```python
from build123d import *

# Parameters (mm, degrees)
F0_W      = 129.2205303907
F0_H      = 41.7168587446
F1_DEPTH  = 152.4
F2_W      = 73.6317485571
F2_H      = 16.954690218
F2_W_2    = 73.8739818335
F2_H_2    = 16.7124718428
F3_DEPTH  = 25.4
F5_DEPTH  = 41.7178587446
F6_W      = 73.389545083
F6_H      = 15.5014246702
F7_DEPTH  = 25.4
F8_W      = 72.4207013845
F8_H      = 15.017002821
F9_DEPTH  = 25.4
F11_DEPTH = 75.7919326425
F13_DEPTH = 105.4396703839
F15_DEPTH = 137.5292986631


with BuildPart() as f1:
    # F0 (on Front) → F1 (new body)
    with BuildSketch(Plane.XZ):
        with Locations((-0.3052428365, -6.4101442695)):
            Rectangle(F0_W, F0_H)
    extrude(amount=F1_DEPTH)

    # F2 (on face) → F3 (cut)
    with BuildSketch(Plane.XY.offset(14.4482851028)):
        with Locations((1.6954615712, -25.9895175695)):
            Rectangle(F2_W, F2_H)
        with Locations((1.8165782094, -58.0823048949)):
            Rectangle(F2_W_2, F2_H_2)
    extrude(amount=-F3_DEPTH, mode=Mode.SUBTRACT)

    # F4 (on face) → F5 (cut, through all)
    with BuildSketch(Plane.XY.offset(14.4482851028)):
        Polygon((64.3050223589, 0), (0, 0), (64.3050223589, -25.4777166992), align=None)
        Polygon((-64.9155080318, 0), (-64.9155080318, -29.2058624327), (0, 0), align=None)
    extrude(amount=-F5_DEPTH, mode=Mode.SUBTRACT)

    # F6 (on face) → F7 (cut)
    with BuildSketch(Plane.XY.offset(14.4482851028)):
        with Locations((1.5743598342, -95.0192883611)):
            Rectangle(F6_W, F6_H)
    extrude(amount=-F7_DEPTH, mode=Mode.SUBTRACT)

    # F8 (on face) → F9 (cut)
    with BuildSketch(Plane.XY.offset(14.4482851028)):
        with Locations((1.0899379849, -126.5065521002)):
            Rectangle(F8_W, F8_H)
    extrude(amount=-F9_DEPTH, mode=Mode.SUBTRACT)

    # F10 (on face) → F11 (cut)
    with BuildSketch(Plane.XY.offset(14.4482851028)):
        Polygon((64.3050223589, -25.4777166992), (50.9865237329, -20.2009137), (50.9865237329, -152.4), align=None)
        Polygon((64.3050223589, -25.4777166992), (50.9865237329, -152.4), (64.3050223589, -152.4), align=None)
    extrude(amount=-F11_DEPTH, mode=Mode.SUBTRACT)

    # F12 (on face) → F13 (cut)
    with BuildSketch(Plane.XY.offset(14.4482851028)):
        Polygon((-45.9601895189, -152.4), (-45.9601895189, -20.677755026), (-64.9155080318, -29.2058624327), (-64.9155080318, -152.4), align=None)
    extrude(amount=-F13_DEPTH, mode=Mode.SUBTRACT)

    # F14 (on face) → F15 (cut)
    with BuildSketch(Plane.XY.offset(14.4482851028)):
        Polygon((0, 0), (-22.9800947595, -10.338877513), (25.4932618665, -10.338877513), align=None)
    extrude(amount=-F15_DEPTH, mode=Mode.SUBTRACT)


solid = f1.part
```
Model file for the job. Use its own axes, mm. A direction names the side the tool comes from. Round coordinates to 2 decimals unless told otherwise and drop trailing zeros. Write each loop counter-clockwise with the first axis right and the second up, starting at its lowest first coordinate (ties: lowest second). Pieces come first, ordered by that corner, then holes. Notation, with made-up numbers: (73.25, 28) - (111.25, 28) arc R14 ccw to (111.25, 39) - close; hole circle Ø3 at (-18.5, 49.25). An arc over 180 degrees is marked (long way). Use CSV: the item, a comma, the result in double quotes. Start each with the question number.
Item 1: Band-saw the part on A-A (z = -3). Write the cut outline in (x, y), and give its area (3 significant figures).
Item 2: Drill centre lines: L1, parallel to Y at x = -7.5, z = -1; L2, parallel to Y at x = -27, z = -6; L3, parallel to X at y = -24, z = 11.5. Where is each one in solid material? Low to high. Write a range as [from, to].
Item 3: Pin check, flat tips, straight feed: P1, Ø12, axis at x = -8, y = -126, coming from the +Z side; P2, Ø12.5, axis at x = 2.5, z = 4, coming from the +Y side; P3, Ø10, axis at x = 10, z = -6.5, coming from the +Y side. Stop position of each tip, or through.
Item 4: Band-saw the part on B-B (x = 20). Write the cut outline in (y, z).
Item 5: Band-saw the part on D-D (y = -92). Write the cut outline in (x, z).
Item 6: Tool access for faces 4 (the face through (37.3, -127, 2)), 5 (the face through (-34.63, -15.58, -6.12)), 6 (the face through (1, -10.339, -6)): list every direction of +Z, -Z, +X, -X, +Y, -Y with a clear straight run to the whole face (end or side of a thin tool).
Item 7: Band-saw the part on C-C (z = -14). Write the cut outline in (x, y).
Item 8: Two-plate mould, pull along Y, no slides. Class faces 1 (the face through (25.14, -9.96, -6.12)), 2 (the face through (1, -102.77, 2)), 3 (the face through (2, -152.4, -6)): released by +Y, released by -Y, zero draft, split by the parting line, or undercut.
Checked values:
1,outline,"(-45.96, -152.4) - (50.99, -152.4) - (50.99, -20.2) - (0, 0) - (25.49, -10.34) - (-22.98, -10.34) - (-45.96, -20.68) - close; hole (-35.12, -134.02) - (37.3, -134.02) - (37.3, -119) - (-35.12, -119) - close; hole (-35.12, -102.77) - (38.27, -102.77) - (38.27, -87.27) - (-35.12, -87.27) - close; hole (-35.12, -66.44) - (38.75, -66.44) - (38.75, -49.73) - (-35.12, -49.73) - close; hole (-35.12, -34.47) - (38.51, -34.47) - (38.51, -17.51) - (-35.12, -17.51) - close"
1,area,"8,830 mm²"
2,L1,"y = [-152.4, -134.02], [-119, -102.77], [-87.27, -66.44], [-49.73, -34.47], [-17.51, -10.34]"
2,L2,"y = [-152.4, -134.02], [-119, -102.77], [-87.27, -66.44], [-49.73, -34.47], [-17.51, -12.15]"
2,L3,"x = [-45.96, -35.12], [38.51, 50.99]"
3,P1,"stops at z = -10.95"
3,P2,"stops at y = 0"
3,P3,"stops at y = -1.98"
4,outline,"(-152.4, -27.27) - (-10.34, -27.27) - (-10.34, 14.45) - (-17.51, 14.45) - (-17.51, -10.95) - (-34.47, -10.95) - (-34.47, 14.45) - (-49.73, 14.45) - (-49.73, -10.95) - (-66.44, -10.95) - (-66.44, 14.45) - (-87.27, 14.45) - (-87.27, -10.95) - (-102.77, -10.95) - (-102.77, 14.45) - (-119, 14.45) - (-119, -10.95) - (-134.02, -10.95) - (-134.02, 14.45) - (-152.4, 14.45) - close; (-8.11, -27.27) - (-7.92, -27.27) - (-7.92, 14.45) - (-8.11, 14.45) - close"
5,outline,"(-45.96, -27.27) - (50.99, -27.27) - (50.99, 14.45) - (38.27, 14.45) - (38.27, -10.95) - (-35.12, -10.95) - (-35.12, 14.45) - (-45.96, 14.45) - close"
6,face 4,"+Z"
6,face 5,"+Z, -Z, -X, +Y"
6,face 6,"+Z, -Z, -X"
7,outline,"(-45.96, -152.4) - (50.99, -152.4) - (50.99, -20.2) - (0, 0) - (25.49, -10.34) - (-22.98, -10.34) - (-45.96, -20.68) - close"
8,face 1,"released by +Y"
8,face 2,"undercut"
8,face 3,"released by -Y"
